from build123d import *

# Parameters (mm, degrees)
SKETCH1_W           = 133.35
SKETCH1_H           = 50.8
BOSS_EXTRUDE1_DEPTH = 3.175
CUT_EXTRUDE1_DEPTH  = 3.175
SKETCH4_W           = 76.2
SKETCH4_H           = 3.175
BOSS_EXTRUDE2_DEPTH = 134.62
SKETCH5_W           = 3.175
SKETCH5_H           = 76.2
BOSS_EXTRUDE3_DEPTH = 127
FILLET1_R           = 38.1
SKETCH6_R           = 14.2875
SKETCH6_R_2         = 3.175
CUT_EXTRUDE3_DEPTH  = 232.059738812
SKETCH3_R           = 3.175
CUT_EXTRUDE2_DEPTH  = 214.036585238


with BuildPart() as part:
    # Sketch1 → Boss-Extrude1 (new body)
    with BuildSketch(Plane(origin=(0, 0, 0), x_dir=(1, 0, 0), z_dir=(0, 1, 0))):
        Rectangle(SKETCH1_W, SKETCH1_H)
    extrude(amount=BOSS_EXTRUDE1_DEPTH)

    # Sketch2 → Cut-Extrude1 (cut)
    with BuildSketch(Plane(origin=(0, 3.175, 0), x_dir=(1, 0, 0), z_dir=(0, 1, 0))):
        with BuildLine():
            Line((-47.625, -12.722), (-38.1, -12.722))
            ThreePointArc((-38.1, -12.722), (-36.322, -14.5), (-38.1, -16.278))
            Line((-38.1, -16.278), (-47.625, -16.278))
            ThreePointArc((-47.625, -16.278), (-49.403, -14.5), (-47.625, -12.722))
        make_face()
        with BuildLine():
            Line((-38.1, 12.722), (-47.625, 12.722))
            ThreePointArc((-47.625, 12.722), (-49.403, 14.5), (-47.625, 16.278))
            Line((-47.625, 16.278), (-38.1, 16.278))
            ThreePointArc((-38.1, 16.278), (-36.322, 14.5), (-38.1, 12.722))
        make_face()
        with BuildLine():
            Line((-38.1, -9.525), (-47.625, -9.525))
            ThreePointArc((-47.625, -9.525), (-57.15, 0), (-47.625, 9.525))
            Line((-47.625, 9.525), (-38.1, 9.525))
            ThreePointArc((-38.1, 9.525), (-28.575, 0), (-38.1, -9.525))
        make_face()
    cut_extrude1 = extrude(amount=-CUT_EXTRUDE1_DEPTH, mode=Mode.SUBTRACT)

    # Mirror1: Cut-Extrude1 across plane
    add(cut_extrude1.mirror(Plane(origin=(0, 0, 0), x_dir=(0, 0, 1), z_dir=(1, 0, 0))), mode=Mode.SUBTRACT)

    # Sketch4 → Boss-Extrude2 (add)
    with BuildSketch(Plane.XY.offset(25.4)):
        with Locations((0, 1.5875)):
            Rectangle(SKETCH4_W, SKETCH4_H)
    extrude(amount=BOSS_EXTRUDE2_DEPTH)

    # Sketch5 → Boss-Extrude3 (add)
    with BuildSketch(Plane.XZ):
        with Locations((39.6875, 121.92)):
            Rectangle(SKETCH5_W, SKETCH5_H)
        with Locations((-39.6875, 121.92)):
            Rectangle(SKETCH5_W, SKETCH5_H)
    extrude(amount=-BOSS_EXTRUDE3_DEPTH)

    # Fillet1
    fillet1_edges = [part.edges().sort_by_distance(p)[0] for p in [
        (39.6875, 127, 160.02),
        (-39.6875, 127, 160.02),
        (39.6875, 127, 83.82),
        (-39.6875, 127, 83.82),
    ]]
    fillet(fillet1_edges, radius=FILLET1_R - 0.0001)  # a hair under: the kernel refuses the full size

    # Sketch6 → Cut-Extrude3 (cut, through all)
    with BuildSketch(Plane.ZY.offset(41.275)):
        with Locations((121.92, 95.25)):
            Circle(SKETCH6_R)
        with Locations((121.92, 50.8)):
            Circle(SKETCH6_R_2)
    extrude(amount=-CUT_EXTRUDE3_DEPTH, mode=Mode.SUBTRACT)

    # Sketch3 → Cut-Extrude2 (cut, through all)
    with BuildSketch(Plane(origin=(0, 3.175, 0), x_dir=(1, 0, 0), z_dir=(0, 1, 0))):
        with Locations(Location((0, 0, 0), (0, 0, 270))):
            Circle(SKETCH3_R)
        with Locations(Location((0, -44.873333333, 0), (0, 0, 270))):
            Circle(SKETCH3_R)
        with Locations(Location((0, -89.746666667, 0), (0, 0, 270))):
            Circle(SKETCH3_R)
        with Locations(Location((0, -134.62, 0), (0, 0, 270))):
            Circle(SKETCH3_R)
    extrude(amount=-CUT_EXTRUDE2_DEPTH, mode=Mode.SUBTRACT)


solid = part.part
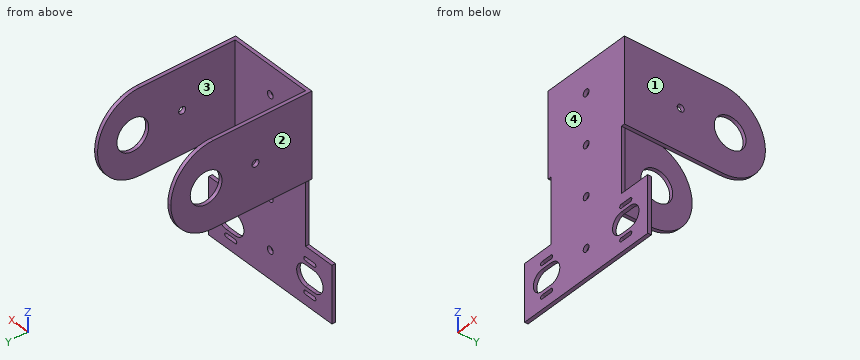
Source: CAD feature listing. Evaluate the final solid. Frame: model axes, mm. Face numbers are marked on the shaded views. Coordinates: 2 decimals unless noted, no trailing zeros. Order: outer loops, then holes, each group sorted by start corner. A loop starts at its lowest first (then second) coordinate and runs counter-clockwise, first axis right, second up. Notation, with made-up numbers: M -37,-23 L -30,-23 A17 ccw -30,-16 Z; hole C 62,-5 d11. An arc over 180 degrees is marked long. Write each question's results on one line, items separated by ' | '. Start each with the question number.
1. Pin query (flat end, axial travel): pin 1 (1 mm diameter, centred on x = 42, y = 2.5, fed in from +Z); pin 2 (23 mm diameter, centred on y = 49, z = 127.5, fed in from -X) (3 decimals); pin 3 (1 mm diameter, centred on x = -41.5, y = 2, fed in from +Z); pin 4 (2 mm diameter, centred on x = 4.5, z = 67, fed in from +Y) (3 decimals). Return the tip coordinate at first contact, or that it passes through.
2. Material intervals for L1, parallel to Y at x = 39.75, z = 121.92 (1 decimal); L2, parallel to Y at x = -18, z = 22 (3 decimals); L3, parallel to X at y = 33.5, z = 116.5 (3 decimals), sorted ascending.
3. Section B-B, the plane x = -45. Return the cut outline in (y, z) (3 decimals).
4. Section D-D, the plane x = 0. Return the cut outline in (y, z) (3 decimals).
5. Section A-A, the plane z = 0. Return the cut outline in (x, y) (3 decimals).
6. Draft query along X for the marked faces 1, 2, 3 and 4. Return one class per face: +X half, -X half, draft (parallel to the pull), parting line (faces both ways), or undercut.
7. Section C-C, the plane y = 76. Return the cut outline in (x, z) (3 decimals).
Solution:
1) pin 1: z = 25.4 | pin 2: x = -41.275 | pin 3: z = 160.02 | pin 4: y = 3.175
2) L1: 0 to 47.6, 54 to 81, 109.5 to 127 | L2: 0 to 3.175 | L3: -41.275 to -38.1, 38.1 to 41.275
3) outline: M 0,-25.4 L 3.175,-25.4 L 3.175,-16.278 L 0,-16.278 Z; M 0,-12.722 L 3.175,-12.722 L 3.175,-9.525 L 0,-9.525 Z; M 0,9.525 L 3.175,9.525 L 3.175,12.722 L 0,12.722 Z; M 0,16.278 L 3.175,16.278 L 3.175,25.4 L 0,25.4 Z
4) outline: M 0,-25.4 L 3.175,-25.4 L 3.175,-3.175 L 0,-3.175 Z; M 0,3.175 L 3.175,3.175 L 3.175,41.698 L 0,41.698 Z; M 0,48.048 L 3.175,48.048 L 3.175,86.572 L 0,86.572 Z; M 0,92.922 L 3.175,92.922 L 3.175,131.445 L 0,131.445 Z; M 0,137.795 L 3.175,137.795 L 3.175,160.02 L 0,160.02 Z
5) outline: M -66.675,0 L -57.15,0 L -57.15,3.175 L -66.675,3.175 Z; M -28.575,0 L -3.175,0 L -3.175,3.175 L -28.575,3.175 Z; M 3.175,0 L 28.575,0 L 28.575,3.175 L 3.175,3.175 Z; M 57.15,0 L 66.675,0 L 66.675,3.175 L 57.15,3.175 Z
6) face 1: +X half | face 2: -X half | face 3: undercut | face 4: draft
7) outline: M -41.275,83.82 L -38.1,83.82 L -38.1,160.02 L -41.275,160.02 Z; M 38.1,83.82 L 41.275,83.82 L 41.275,160.02 L 38.1,160.02 Z
